```python
from build123d import *

# Parameters (mm, degrees)
SKETCH1_W                                       = 40
SKETCH1_H                                       = 37.5
BOSS_EXTRUDE1_DEPTH                             = 5
SKETCH2_W                                       = 40
SKETCH2_H                                       = 30
BOSS_EXTRUDE2_DEPTH                             = 8
BOSS_EXTRUDE3_DEPTH                             = 5
BOSS_EXTRUDE4_START                             = -40
BOSS_EXTRUDE4_DEPTH                             = 5
CSK_FOR_M3_FLAT_HEAD_MACHINE_SCREW1_D           = 3.4
CSK_FOR_M3_FLAT_HEAD_MACHINE_SCREW1_DEPTH       = 6
CSK_FOR_M3_FLAT_HEAD_MACHINE_SCREW1_CSINK_D     = 6.3
CSK_FOR_M3_FLAT_HEAD_MACHINE_SCREW1_CSINK_ANGLE = 90
CSK_FOR_M3_FLAT_HEAD_MACHINE_SCREW1_TIP         = 1.021463052
F_12_0_12_DIAMETER_HOLE1_D                      = 12
F_12_0_12_DIAMETER_HOLE1_DEPTH                  = 6
F_12_0_12_DIAMETER_HOLE1_TIP                    = 3.605163714


with BuildPart() as part:
    # Sketch1 → Boss-Extrude1 (new body)
    with BuildSketch(Plane(origin=(0, 0, 0), x_dir=(1, 0, 0), z_dir=(0, 1, 0))):
        Rectangle(SKETCH1_W, SKETCH1_H)
    extrude(amount=BOSS_EXTRUDE1_DEPTH)

    # Sketch2 → Boss-Extrude2 (add)
    with BuildSketch(Plane.XY.offset(18.75)):
        with Locations((0, 15)):
            Rectangle(SKETCH2_W, SKETCH2_H)
    extrude(amount=-BOSS_EXTRUDE2_DEPTH)

    # Sketch3 → Boss-Extrude3 (add)
    with BuildSketch(Plane(origin=(20, 0, 0), x_dir=(0, 0, -1), z_dir=(1, 0, 0))):
        Polygon((-10.75, 30), (18.75, 5), (-10.75, 5), align=None)
    extrude(amount=-BOSS_EXTRUDE3_DEPTH)

    # Sketch3<2> → Boss-Extrude4 (add)
    with BuildSketch(Plane(origin=(20, 0, 0), x_dir=(0, 0, -1), z_dir=(1, 0, 0)).offset(BOSS_EXTRUDE4_START)):
        Polygon((-10.75, 30), (18.75, 5), (-10.75, 5), align=None)
    extrude(amount=BOSS_EXTRUDE4_DEPTH)

    # CSK for M3 Flat Head Machine Screw1
    with Locations(Plane(origin=(0, 5, 0), x_dir=(1, 0, 0), z_dir=(0, 1, 0))):
        with Locations((8.660254038, -3.5), (0, 11.5), (-8.660254038, -3.5)):
            CounterSinkHole(CSK_FOR_M3_FLAT_HEAD_MACHINE_SCREW1_D / 2, CSK_FOR_M3_FLAT_HEAD_MACHINE_SCREW1_CSINK_D / 2, depth=CSK_FOR_M3_FLAT_HEAD_MACHINE_SCREW1_DEPTH, counter_sink_angle=CSK_FOR_M3_FLAT_HEAD_MACHINE_SCREW1_CSINK_ANGLE)
            with Locations((0, 0, -(CSK_FOR_M3_FLAT_HEAD_MACHINE_SCREW1_DEPTH + CSK_FOR_M3_FLAT_HEAD_MACHINE_SCREW1_TIP / 2))):  # 118° drill point
                Cone(0, CSK_FOR_M3_FLAT_HEAD_MACHINE_SCREW1_D / 2, CSK_FOR_M3_FLAT_HEAD_MACHINE_SCREW1_TIP, mode=Mode.SUBTRACT)

    # Ø12.0 (12) Diameter Hole1
    with Locations(Plane(origin=(0, 0, 10.75), x_dir=(-1, 0, 0), z_dir=(0, 0, -1))):
        with Locations((0, 17.5)):
            Hole(F_12_0_12_DIAMETER_HOLE1_D / 2, depth=F_12_0_12_DIAMETER_HOLE1_DEPTH)
            with Locations((0, 0, -(F_12_0_12_DIAMETER_HOLE1_DEPTH + F_12_0_12_DIAMETER_HOLE1_TIP / 2))):  # 118° drill point
                Cone(0, F_12_0_12_DIAMETER_HOLE1_D / 2, F_12_0_12_DIAMETER_HOLE1_TIP, mode=Mode.SUBTRACT)


solid = part.part
```
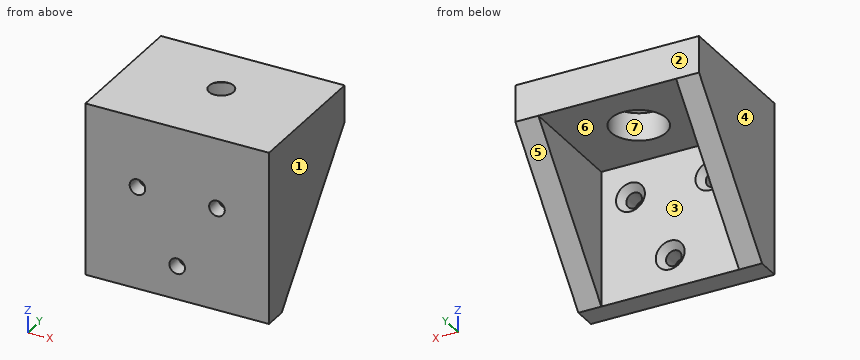
Model file for the job. Use its own axes, mm. Face numbers are marked on the shaded views. A direction names the side the tool comes from. Give positions to 0.01 mm unless a question says otherwise; leave off trailing zeros. Loops run counter-clockwise (first coordinate to the right, second up) from the corner with the lowest first, then second, coordinate; pieces in that order, holes last. Notation, with made-up numbers: (39.5, 47) - (44.5, 47) arc R28 cw to (44.5, 85) - close; hole circle Ø6 at (-1.75, 50). An arc over 180 degrees is marked (long way). One line per item, written item: value. Start each with the question number.
1. Slice it at B-B (x = 0). List the corners of the cut face in (y, z), plus the area to 3 significant figures.
2. Probe L1, parallel to Z at x = 0, y = 1.2; L2, parallel to Y at x = 0, z = 13; L3, parallel to X at y = 15, z = -3. List the from-to ranges inside material, lowest first. Write a range as from..to.
3. Slice it at C-C (y = 17.5). List the corners of the cut face in (x, z).
4. Pin check, flat tips, straight feed: pin 1 (9 mm diameter, centred on x = 0, z = -7, fed in from +Y); pin 2 (5.5 mm diameter, centred on x = 8.66, z = 3.5, fed in from +Y). Stop position of each tip, or through.
5. Which spindle directions (+Z, -Z, +X, -X, +Y, -Y) get a long thin tool onto all of the face, cutting with end or side? Do the marked faces 5, 6 and 7. Say none if no direction does.
6. Pull direction X, two halves, no side cores. Call the marked faces 1, 2, 3 and 4: pulls with the +X half, pulls with the -X half, needs draft (parallel to the pull), parting line crosses it, or undercut.
7. Slice it at D-D (z = 3.5). List the corners of the cut face in (x, y).
8. Slice it at A-A (z = 14.5). List the corners of the cut face in (x, y), plus the area to 3 significant figures.
Solution:
1. outline: (0, -18.75) - (5, -18.75) - (5, -14.65) - (3.55, -13.2) - (0, -13.2) - close; (0, -9.8) - (3.55, -9.8) - (5, -8.35) - (5, 10.75) - (11.5, 10.75) - (11.5, 16.75) - (14.83, 18.75) - (0, 18.75) - close; (20.17, 18.75) - (23.5, 16.75) - (23.5, 10.75) - (30, 10.75) - (30, 18.75) - close
1. area: 279 mm^2
2. L1: z = -18.75..-13.2, -9.8..18.75
2. L2: y = 0..11.5, 23.5..30
2. L3: x = -20..-15, 15..20
3. outline: (-20, -4) - (-15, -4) - (-15, 10.75) - (-6, 10.75) - (-6, 16.75) - (-2.67, 18.75) - (-20, 18.75) - close; (2.67, 18.75) - (6, 16.75) - (6, 10.75) - (15, 10.75) - (15, -4) - (20, -4) - (20, 18.75) - close
4. pin 1: stops at y = 5
4. pin 2: stops at y = 4.6
5. face 5: -Z, +X, -X, +Y
5. face 6: -Z, +Y
5. face 7: -Z
6. face 1: pulls with the +X half
6. face 2: needs draft
6. face 3: undercut
6. face 4: pulls with the -X half
7. outline: (-20, 0) - (-10.36, 0) - (-10.36, 3.55) - (-11.81, 5) - (-15, 5) - (-15, 23.86) - (-20, 23.86) - close; (-6.96, 0) - (6.96, 0) - (6.96, 3.55) - (5.51, 5) - (-5.51, 5) - (-6.96, 3.55) - close; (10.36, 0) - (20, 0) - (20, 23.86) - (15, 23.86) - (15, 5) - (11.81, 5) - (10.36, 3.55) - close
8. outline: (-20, 0) - (20, 0) - (20, 30) - (-20, 30) - close; hole circle Ø12 at (0, 17.5)
8. area: 1,090 mm^2
